Work out the finished part from the listing and answer in its coordinate system (mm). A direction names the side the tool comes from. Round coordinates to 2 decimals unless told otherwise and drop trailing zeros. Loops run counter-clockwise (first coordinate to the right, second up) from the corner with the lowest first, then second, coordinate; pieces in that order, holes last. Notation, with made-up numbers: (74.5, -1) -> (91.5, -1) arc R9 cw to (91.5, 7) -> close; hole circle Ø9 at (79, 23.5). An arc over 180 degrees is marked (long way). Use one line per item in the form item = value.
```python
from build123d import *

# Parameters (mm, degrees)
BOSS_EXTRUDE1_DEPTH   = 5
CUT_EXTRUDE1_REACH    = 84.998
CUT_EXTRUDE2_DEPTH    = 9
SKETCH7_W             = 26.5
SKETCH7_H             = 10.5
CUT_EXTRUDE3_DEPTH    = 0.7
CUT_EXTRUDE4_DEPTH    = 1.5
F_4_0MM_DOWEL_HOLE1_D = 4.5
CUT_EXTRUDE6_DEPTH    = 2
CHAMFER1_SIZE         = 1
SKETCH12_W            = 4
SKETCH12_H            = 16
CUT_EXTRUDE5_DEPTH    = 0.7
SKETCH13_W            = 7.3
SKETCH13_H            = 6.5
BOSS_EXTRUDE2_DEPTH   = 0.2
FILLET1_R             = 1


with BuildPart() as part:
    # Sketch1 → Boss-Extrude1 (new body)
    with BuildSketch(Plane(origin=(0, 0, 0), x_dir=(1, 0, 0), z_dir=(0, 1, 0))):
        Polygon((0, -4), (0, 4), (6.593945807, 6.4), (82.6, 6.4), (82.6, -6.4), (6.593945807, -6.4), align=None)
    extrude(amount=-BOSS_EXTRUDE1_DEPTH)

    # Sketch2 → Cut-Extrude1 (cut, up to next)
    with BuildSketch(Plane(origin=(0, 0, 0), x_dir=(1, 0, 0), z_dir=(0, 1, 0)), mode=Mode.PRIVATE) as cut_extrude1_sk1:
        with BuildLine():
            Line((62.85, 2.25), (77.85, 2.25))
            ThreePointArc((77.85, 2.25), (80.1, 0), (77.85, -2.25))
            Line((77.85, -2.25), (62.85, -2.25))
            ThreePointArc((62.85, -2.25), (60.6, 0), (62.85, 2.25))
        make_face()
    cut_extrude1_tool1 = extrude(cut_extrude1_sk1.sketch, amount=-CUT_EXTRUDE1_REACH, mode=Mode.PRIVATE) & part.part
    # Sketch2 → Cut-Extrude1 (cut, up to next)
    with BuildSketch(Plane(origin=(0, 0, 0), x_dir=(1, 0, 0), z_dir=(0, 1, 0)), mode=Mode.PRIVATE) as cut_extrude1_sk2:
        with BuildLine():
            Line((52.85, -2.25), (37.85, -2.25))
            ThreePointArc((37.85, -2.25), (35.6, 0), (37.85, 2.25))
            Line((37.85, 2.25), (52.85, 2.25))
            ThreePointArc((52.85, 2.25), (55.1, 0), (52.85, -2.25))
        make_face()
    cut_extrude1_tool2 = extrude(cut_extrude1_sk2.sketch, amount=-CUT_EXTRUDE1_REACH, mode=Mode.PRIVATE) & part.part
    add(cut_extrude1_tool1.solids().sort_by_distance((70.35, 0, 0))[0], mode=Mode.SUBTRACT)
    add(cut_extrude1_tool2.solids().sort_by_distance((45.35, 0, 0))[0], mode=Mode.SUBTRACT)

    # Sketch6 → Cut-Extrude2 (cut, symmetric)
    with BuildSketch(Plane.XY):
        Polygon((0, -3.2), (10.208307275, -5), (0, -5), align=None)
    extrude(amount=CUT_EXTRUDE2_DEPTH, both=True, mode=Mode.SUBTRACT)

    # Sketch7 → Cut-Extrude3 (cut)
    with BuildSketch(Plane(origin=(0, 0, 0), x_dir=(1, 0, 0), z_dir=(0, 1, 0))):
        with Locations((13.25, 0)):
            Rectangle(SKETCH7_W, SKETCH7_H)
    extrude(amount=-CUT_EXTRUDE3_DEPTH, mode=Mode.SUBTRACT)

    # Sketch8 → Cut-Extrude4 (cut)
    with BuildSketch(Plane(origin=(0, -0.7, 0), x_dir=(1, 0, 0), z_dir=(0, 1, 0))):
        with BuildLine():
            Line((0, -3.1), (0, 3.1))
            Line((0, 3.1), (3, 3.1))
            ThreePointArc((3, 3.1), (4, 2.1), (3, 1.1))
            Line((3, 1.1), (3, 0))
            Line((3, 0), (3, -1.1))
            ThreePointArc((3, -1.1), (4, -2.1), (3, -3.1))
            Line((3, -3.1), (0, -3.1))
        make_face()
    extrude(amount=-CUT_EXTRUDE4_DEPTH, mode=Mode.SUBTRACT)

    # Ø4.0mm Dowel Hole1 (through all)
    with Locations(Plane(origin=(0, -0.7, 0), x_dir=(1, 0, 0), z_dir=(0, 1, 0))):
        with Locations((12.5, 0)):
            Hole(F_4_0MM_DOWEL_HOLE1_D / 2)

    # Sketch14 → Cut-Extrude6 (cut)
    with BuildSketch(Plane.XZ.offset(5)):
        Polygon((16, -2.020725942), (16, 2.020725942), (12.5, 4.041451884), (9, 2.020725942), (9, -2.020725942), (12.5, -4.041451884), align=None)
    extrude(amount=-CUT_EXTRUDE6_DEPTH, mode=Mode.SUBTRACT)

    # Chamfer1
    chamfer1_edges = [part.edges().sort_by_distance(p)[0] for p in [
        (82.6, -2.5, -6.4),
        (82.6, -2.5, 6.4),
    ]]
    chamfer(chamfer1_edges, length=CHAMFER1_SIZE)

    # Sketch12 → Cut-Extrude5 (cut)
    with BuildSketch(Plane(origin=(0, 0, 0), x_dir=(1, 0, 0), z_dir=(0, 1, 0))):
        with Locations((2, 0)):
            Rectangle(SKETCH12_W, SKETCH12_H)
    extrude(amount=-CUT_EXTRUDE5_DEPTH, mode=Mode.SUBTRACT)

    # Sketch13 → Boss-Extrude2 (add)
    with BuildSketch(Plane(origin=(0, -0.7, 0), x_dir=(1, 0, 0), z_dir=(0, 1, 0))):
        with Locations((22.85, 0)):
            Rectangle(SKETCH13_W, SKETCH13_H)
    extrude(amount=BOSS_EXTRUDE2_DEPTH)

    # Fillet1
    fillet1_edges = [part.edges().sort_by_distance(p)[0] for p in [
        (26.5, -0.35, 5.25),
        (26.5, -0.6, 3.25),
        (26.5, -0.6, -3.25),
        (26.5, -0.35, -5.25),
    ]]
    fillet(fillet1_edges, radius=FILLET1_R - 0.0001)  # a hair under: the kernel refuses the full size


solid = part.part
```
(1) For faces 1 (the flat face through (1, -1, -3.1)), 2 (the flat face through (70, -2, 2.25)), 3 (the flat face through (0, -2.5, 0.1)), 4 (the flat face through (9, -4, 0)), 5 (the flat face through (4.076, -2.151, 5.483)), determine the directions among +Z, -Z, +X, -X, +Y, -Y from which every point of the face is accessible in a straight line to the end or side of a thin tool.
Completed:
face_1 = -X, +Y
face_2 = +Y, -Y
face_3 = +Z, -Z, -X, +Y, -Y
face_4 = -Y
face_5 = +Z, -X, +Y, -Y
(2) Given P1, Ø3.5, axis at x = 13.5, z = -1, coming from the -Y side; P2, Ø5, axis at x = 19, z = -0.5, coming from the +Y side; P3, Ø1.2, axis at x = 2.5, z = -0.5, coming from the +Y side, each flat-ended and moving along its own axis, determine where each tip first touches the part or whether it passes through.
Completed:
P1 = -3
P2 = -0.5
P3 = -0.7
(3) Consider L1, parallel to X at y = -2.8, z = 0.25; L2, parallel to Z at x = 12.5, y = -2; L3, parallel to X at y = -2.5, z = 1. Determine where each line is inside the solid, lowest interval first.
Completed:
L1 = 0 to 10.26, 14.74 to 35.61, 55.09 to 60.61, 80.09 to 82.6
L2 = -6.4 to -2.25, 2.25 to 6.4
L3 = 0 to 10.48, 14.52 to 35.83, 54.87 to 60.83, 79.87 to 82.6
(4) Find section A-A, the plane x = 43. Write down the section's boundary in (y, z).
Completed:
outline = (-5, -6.4) -> (0, -6.4) -> (0, -2.25) -> (-5, -2.25) -> close; (-5, 2.25) -> (0, 2.25) -> (0, 6.4) -> (-5, 6.4) -> close
(5) For a pull along Z with two mould halves and no side action, classify faces 6 (the flat face through (47, -5, -3)), 7 (the flat face through (45, -2, 6.4)), 8 (the flat face through (44, -2, -6.4)), 9 (the flat face through (2, -2.2, 0)) as +Z half, -Z half, draft (parallel to the pull), parting line (faces both ways), or undercut.
Completed:
face_6 = draft
face_7 = +Z half
face_8 = -Z half
face_9 = undercut
